Design review of the part built by this model. Coordinates are the model's own, in mm. Give positions to 0.01 mm unless a question says otherwise; leave off trailing zeros. Write each loop counter-clockwise with the first axis right and the second up, starting at its lowest first coordinate (ties: lowest second). Pieces come first, ordered by that corner, then holes. Notation, with made-up numbers: (11.25, 85.25) -> (63.25, 85.25) arc R18 cw to (63.25, 100.25) -> close; hole circle Ø11 at (38, -38). An arc over 180 degrees is marked (long way). Write each question's results on one line, items separated by ' | '. Start each with the question number.
(1) Clearance check with flat-ended pins moving along their axes: pin 1 (1 mm diameter, centred on y = -2, z = 54.5, fed in from +X); pin 2 (5 mm diameter, centred on y = -1.5, z = 71.5, fed in from -X). State where each tip first meets the part, or that it passes through.
(2) Take a section at A-A (z = 61). State the section outline as (x, y) points, plus the area to 3 significant figures.
(3) To check wall thickness, follow probe 1 along Z at (x, y) = (-2.25, -3.25); probe 2 along Y at (x, z) = (0, 18.5); probe 3 along Z at (x, y) = (0.75, -2.75). State the ranges of each line that lie inside material, in increasing order.
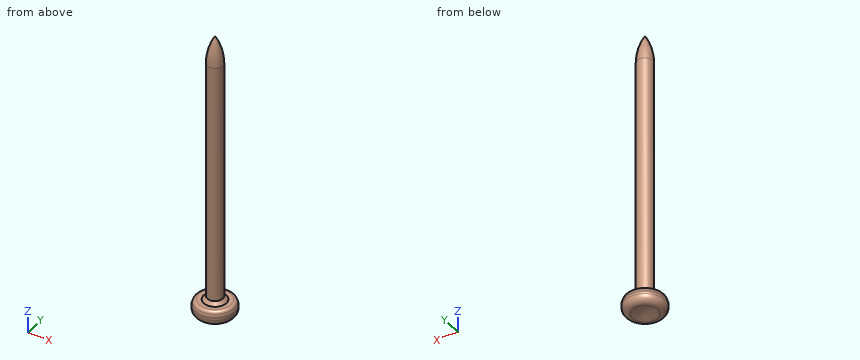
from build123d import *


with BuildPart() as part:
    # Skizze1 → Rotation1 (revolve)
    with BuildSketch(Plane(origin=(0, 0, 0), x_dir=(0, 0, -1), z_dir=(1, 0, 0)), mode=Mode.PRIVATE) as rotation1_sk:
        with BuildLine():
            Line((-0.006814835, 3.47456669), (-0.937822174, 0))
            Line((-0.937822174, 0), (-82, 0))
            ThreePointArc((-82, 0), (-78.155192535, 1.676795679), (-74, 2.25))
            Line((-74, 2.25), (-5.3, 2.25))
            Line((-5.3, 2.25), (-4.3, 3.25))
            Line((-4.3, 3.25), (-4.3, 4.52924078))
            ThreePointArc((-4.3, 4.52924078), (-4.111242185, 5.113951065), (-3.616227766, 5.477924078))
            Line((-3.616227766, 5.477924078), (-2.953950106, 5.698683298))
            ThreePointArc((-2.953950106, 5.698683298), (-2.797904583, 5.737087458), (-2.63772234, 5.75))
            Line((-2.63772234, 5.75), (-2, 5.75))
            ThreePointArc((-2, 5.75), (-0.585786438, 5.164213562), (0, 3.75))
            Line((0, 3.75), (0, 3.5263305))
            ThreePointArc((0, 3.5263305), (-0.001711028, 3.500225261), (-0.006814835, 3.47456669))
        make_face()
    revolve(rotation1_sk.sketch.rotate(Axis((0, 0, 0), (0, 0, 1)), 90), axis=Axis((0, 0, 0), (0, 0, 1)))  # turned: the seam where the file's is


solid = part.part
Report:
1) pin 1: x = 1.68 | pin 2: x = -2.25
2) outline: circle Ø4.5 at (0, 0) | area: 15.9 mm2
3) probe 1: 0.01 to 4.3 | probe 2: -2.25 to 2.25 | probe 3: 0.17 to 4.7
